```python
from build123d import *

# Parameters (mm, degrees)
ESBO_O1_W                = 19
ESBO_O1_H                = 19
RESSALTO_EXTRUS_O1_DEPTH = 260
CASCA2_T                 = -1
CORTE_EXTRUS_O1_DEPTH    = 20
CORTE_EXTRUS_O3_DEPTH    = 20
ESBO_O5_R                = 1.5
CORTE_EXTRUS_O4_DEPTH    = 52.987151397
ESBO_O7_W                = 19
ESBO_O7_H                = 19
CORTE_EXTRUS_O6_DEPTH    = 52.987151397


with BuildPart() as part:
    # Esboço1 → Ressalto-extrusão1 (new body)
    with BuildSketch(Plane.XY):
        Rectangle(ESBO_O1_W, ESBO_O1_H)
    extrude(amount=RESSALTO_EXTRUS_O1_DEPTH)

    # Casca2
    casca2_openings = [part.faces().sort_by_distance(p)[0] for p in [
        (0, 0, 260),
        (0, 0, 0),
    ]]
    offset(amount=CASCA2_T, openings=casca2_openings, kind=Kind.INTERSECTION)

    # Esboço2 → Corte-extrusão1 (cut, through all)
    with BuildSketch(Plane(origin=(9.5, 0, 0), x_dir=(0, 0, -1), z_dir=(1, 0, 0))):
        Polygon((0, 9.5), (-58.475987206, -9.5), (0, -9.5), align=None)
    extrude(amount=-CORTE_EXTRUS_O1_DEPTH, mode=Mode.SUBTRACT)

    # Esboço4 → Corte-extrusão3 (cut, through all)
    with BuildSketch(Plane(origin=(9.5, 0, 0), x_dir=(0, 0, -1), z_dir=(1, 0, 0))):
        Polygon((-168.550335734, 10.473717073), (-161.289503816, -11.872825786), (-264.812755879, -45.509569399), (-289.05777752, 22.149749677), (-184.516070462, 59.611196004), align=None)
    extrude(amount=-CORTE_EXTRUS_O3_DEPTH, mode=Mode.SUBTRACT)

    # Esboço5 → Corte-extrusão4 (cut, through all)
    with BuildSketch(Plane(origin=(0, 9.5, 0), x_dir=(1, 0, 0), z_dir=(0, 0.951056516, 0.309016994))):
        with Locations((0, -23)):
            Circle(ESBO_O5_R)
        with Locations((0, -48)):
            Circle(ESBO_O5_R)
    extrude(amount=CORTE_EXTRUS_O4_DEPTH, mode=Mode.SUBTRACT)

    # Esboço7 → Corte-extrusão6 (cut, through all)
    with BuildSketch(Plane(origin=(0, 8.592830723, 2.791979948), x_dir=(1, 0, 0), z_dir=(0, -0.951056516, -0.309016994))):
        with Locations((0, 6.564338553)):
            Rectangle(ESBO_O7_W, ESBO_O7_H)
    extrude(amount=-CORTE_EXTRUS_O6_DEPTH, mode=Mode.SUBTRACT)


solid = part.part
```
Geometry: final body of the model. Coordinates: model frame, mm. A direction names the side the tool comes from. Coordinates: 2 decimals unless noted, no trailing zeros. Write each loop counter-clockwise with the first axis right and the second up, starting at its lowest first coordinate (ties: lowest second). Pieces come first, ordered by that corner, then holes. Notation, with made-up numbers: M 72.5,-26 L 122.5,-26 A18 cw 122.5,-1 Z; hole C 6.5,-40 d10. An arc over 180 degrees is marked long. Use CSV: the item, a comma, the result in double quotes. Start each with the question number.
1. Cut plane D-D on z = 37. Return the cut outline in (x, y), plus the area to 3 significant figures.
2. Cut plane A-A on z = 120. Return the cut outline in (x, y).
3. Reachability of faces 5 (the face through (8.5, 0, 92)), 6 (the face through (0, 9.5, 93)) from +Z, -Z, +X, -X, +Y, -Y: full face, straight path, thin tool, end or side. Return the list, or none.
4. Cut plane B-B on y = -7. Return the cut outline in (x, z).
5. Mould query, pull axis X, two halves, no side actions, for faces 1 (the face through (-0.044, 8.725, 19.726)), 2 (the face through (-1.5, 9.01, 50.24)), 3 (the face through (9.5, 0, 92)), 4 (the face through (-9.5, 0, 92)). Classes: pulls with the +X half, pulls with the -X half, needs draft (parallel to the pull), parting line crosses it, or undercut.
6. Ray query, probe 1 along Y at (x, z) = (6.75, 143.5); probe 2 along Y at (x, z) = (-6.75, 25). Return the intervals inside material, ascending.
7. Cut plane C-C on x = 3.75. Return the cut outline in (y, z).
8. First-contact query: P1, Ø3, axis at x = -6.5, y = -6.5, coming from the +Z side. Flat tip, straight axial feed; report the tip coordinate or a pass-through.
Entries:
1,outline,"M -9.5,-2.52 L -8.5,-2.52 L -8.5,8.5 L 8.5,8.5 L 8.5,-2.52 L 9.5,-2.52 L 9.5,9.5 L -9.5,9.5 Z"
1,area,"41.0 mm²"
2,outline,"M -9.5,-9.5 L 9.5,-9.5 L 9.5,9.5 L -9.5,9.5 Z; hole M -8.5,-8.5 L 8.5,-8.5 L 8.5,8.5 L -8.5,8.5 Z"
3,face 5,"+Z, -Z"
3,face 6,"+Z, -Z, +X, -X, +Y"
4,outline,"M -9.5,50.78 L -8.5,50.78 L -8.5,162.87 L -9.5,162.87 Z; M 8.5,50.78 L 9.5,50.78 L 9.5,162.87 L 8.5,162.87 Z"
5,face 1,"needs draft"
5,face 2,"undercut"
5,face 3,"pulls with the +X half"
5,face 4,"pulls with the -X half"
6,probe 1,"-9.5 to -8.5, 8.5 to 9.5"
6,probe 2,"8.5 to 9.5"
7,outline,"M -9.5,58.48 L -8.5,55.4 L -8.5,162.39 L -9.5,162.06 Z; M 8.5,19.65 L 9.5,19.98 L 9.5,168.23 L 8.5,167.91 Z"
8,P1,"through"
